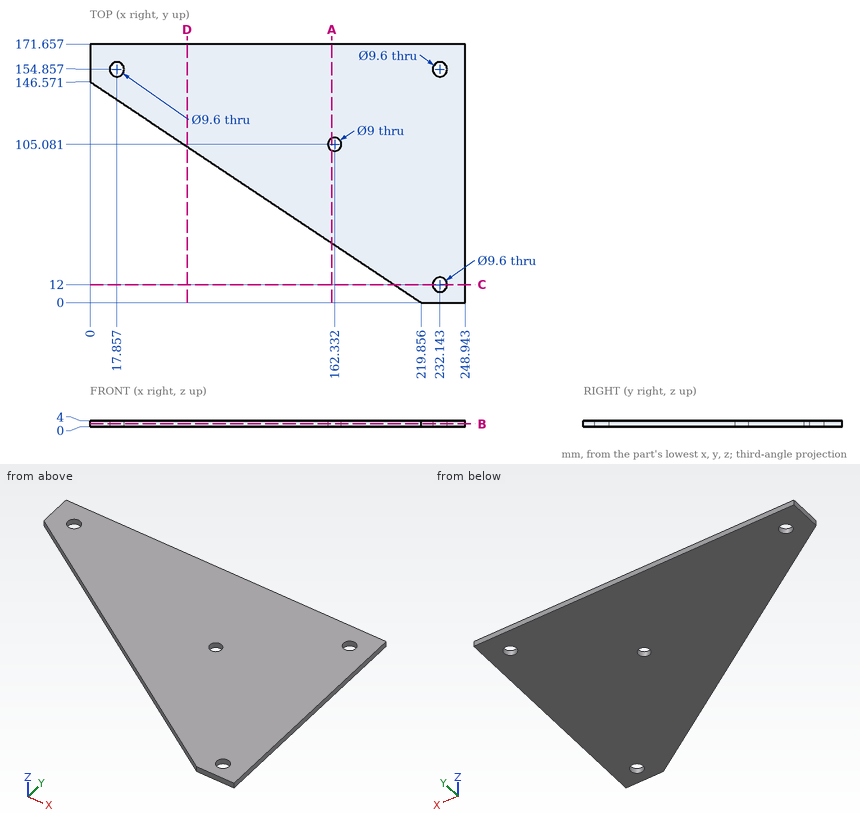
The figure shows three views and two pictorial views of one solid part (mm, origin at its lowest corner). Answer the questions. Round coordinates to 2 decimals unless told otherwise and drop trailing zeros. Loops run counter-clockwise (first coordinate to the right, second up) from the corner with the lowest first, then second, coordinate; pieces in that order, holes last. Notation, with made-up numbers: (80, 52) - (101, 52) arc R34 cw to (101, 87) - close; hole circle Ø6 at (-27.75, 76). An arc over 180 degrees is marked (long way). One line per question, with ' | ' between items. Start each with the question number.
Q1. Find the intervals of material crossed by L1, parallel to X at y = 157, z = 1.55; L2, parallel to Y at x = 165, z = 1.3 (1 decimal); L3, parallel to Y at x = 69, z = 3, in increasing order.
Q2. Section B-B on z = 1.85 is taken. Give the vertices of the cut face in (x, y), plus the area to 3 significant figures.
Q3. Section C-C on y = 12 is taken. Give the vertices of the cut face in (x, z).
Q4. Section D-D on x = 64.5 is taken. Give the vertices of the cut face in (y, z), plus the area to 3 significant figures.
Q5. Section A-A on x = 160.5 is taken. Give the vertices of the cut face in (y, z).
Established:
1) L1: 0 to 13.56, 22.15 to 227.85, 236.44 to 248.94 | L2: 36.6 to 101.5, 108.7 to 171.7 | L3: 100.57 to 171.66
2) outline: (0, 146.57) - (219.86, 0) - (248.94, 0) - (248.94, 171.66) - (0, 171.66) - close; hole circle Ø9.6 at (17.86, 154.86); hole circle Ø9 at (162.33, 105.08); hole circle Ø9.6 at (232.14, 12); hole circle Ø9.6 at (232.14, 154.86) | area: 26,300 mm²
3) outline: (201.86, 0) - (227.34, 0) - (227.34, 4) - (201.86, 4) - close; (236.94, 0) - (248.94, 0) - (248.94, 4) - (236.94, 4) - close
4) outline: (103.57, 0) - (171.66, 0) - (171.66, 4) - (103.57, 4) - close | area: 272 mm²
5) outline: (39.57, 0) - (100.97, 0) - (100.97, 4) - (39.57, 4) - close; (109.19, 0) - (171.66, 0) - (171.66, 4) - (109.19, 4) - close
